The model under review builds one solid part; all positions refer to its coordinate system, in mm. A direction names the side the tool comes from. Round coordinates to 2 decimals unless told otherwise and drop trailing zeros. Order: outer loops, then holes, each group sorted by start corner. A loop starts at its lowest first (then second) coordinate and runs counter-clockwise, first axis right, second up. Notation, with made-up numbers: (-6.75, 3) -> (8.25, 3) arc R30 ccw to (8.25, 29) -> close; hole circle Ø5 at (-26, 78.5). An arc over 180 degrees is marked (long way). Use a Markdown table: item, result. Add a question column.
```python
from build123d import *

# Parameters (mm, degrees)
F1_DEPTH = 25


with BuildPart() as f1:
    # F0 (on Front) → F1 (new body)
    with BuildSketch(Plane.XZ):
        Polygon((-21.796276, -30), (21.796276, -30), (35.267115, 11.45898), (0, 37.082039), (-35.267115, 11.45898), align=None)
        Polygon((-17.320508, 0), (-8.660254, 15), (8.660254, 15), (17.320508, 0), (8.660254, -15), (-8.660254, -15), align=None, mode=Mode.SUBTRACT)
    extrude(amount=F1_DEPTH)


solid = f1.part
```
Q1. To check wall thickness, follow line 1 along Z through (x, y) = (5.5, -6.5); line 2 along X through (y, z) = (-22.5, -3.5); line 3 along Z through (x, y) = (-16, -23.5). State the ranges of each line that lie inside material, in increasing order.
Q2. Add section A-A, the plane x = -12. Give the boundary of the cut face in (y, z).
Q3. Add section B-B, the plane y = -16.25. Give the boundary of the cut face in (x, z), then the cut area to 3 significant figures.
Q4. For faces 1 (the face through (15.2, -25, 4)), 2 (the face through (0, -12, -15)), list the 3-axis set-ups (+Z, -Z, +X, -X, +Y, -Y) from which the entire face can be reached by the end or side of a thin tool; tool diameter is ignored.
Q5. For pin 1 (3 mm diameter, centred on y = -19, z = 2, fed in from +X); pin 2 (3 mm diameter, centred on x = 15, y = -3, fed in from +Z); pin 3 (5 mm diameter, centred on y = -11, z = 11.5, fed in from -X), all flat-tipped, find the tip position at first contact; note any pin that passes through.
Q6. Add section D-D, the plane z = 28. Give the boundary of the cut face in (x, y), then the cut area to 3 significant figures.
Q7. Draft analysis for pull direction Z (two halves, no side actions). For faces 3 (the face through (13.05, -12.32, -7.4)), 4 (the face through (12.93, -12.325, 7.605)), 5 (the face through (-28.626, -12.325, -8.98)), 6 (the face through (-17.387, -12.325, 24.45)), state which applies: released by +Z, released by -Z, zero draft, split by the parting line, or undercut.
Q8. Add section C-C, the plane z = -6. Give the boundary of the cut face in (x, y), then the cut area to 3 significant figures.
Return value:
| question | item | result |
|---|---|---|
| 1 | line 1 | -30 to -15, 15 to 33.09 |
| 1 | line 2 | -30.41 to -15.3, 15.3 to 30.41 |
| 1 | line 3 | -30 to -2.29, 2.29 to 25.46 |
| 2 | outline | (-25, -30) -> (0, -30) -> (0, -9.22) -> (-25, -9.22) -> close; (-25, 9.22) -> (0, 9.22) -> (0, 28.36) -> (-25, 28.36) -> close |
| 3 | outline | (-35.27, 11.46) -> (-21.8, -30) -> (21.8, -30) -> (35.27, 11.46) -> (0, 37.08) -> close; hole (-17.32, 0) -> (-8.66, -15) -> (8.66, -15) -> (17.32, 0) -> (8.66, 15) -> (-8.66, 15) -> close |
| 3 | area | 2,490 mm² |
| 4 | face 1 | +Z, -Z, +X, -X, -Y |
| 4 | face 2 | +Y, -Y |
| 5 | pin 1 | x = 32.68 |
| 5 | pin 2 | z = 27.27 |
| 5 | pin 3 | x = -35.27 |
| 6 | outline | (-12.5, -25) -> (12.5, -25) -> (12.5, 0) -> (-12.5, 0) -> close |
| 6 | area | 625 mm² |
| 7 | face 3 | undercut |
| 7 | face 4 | undercut |
| 7 | face 5 | released by -Z |
| 7 | face 6 | released by +Z |
| 8 | outline | (-29.59, -25) -> (-13.86, -25) -> (-13.86, 0) -> (-29.59, 0) -> close; (13.86, -25) -> (29.59, -25) -> (29.59, 0) -> (13.86, 0) -> close |
| 8 | area | 787 mm² |
